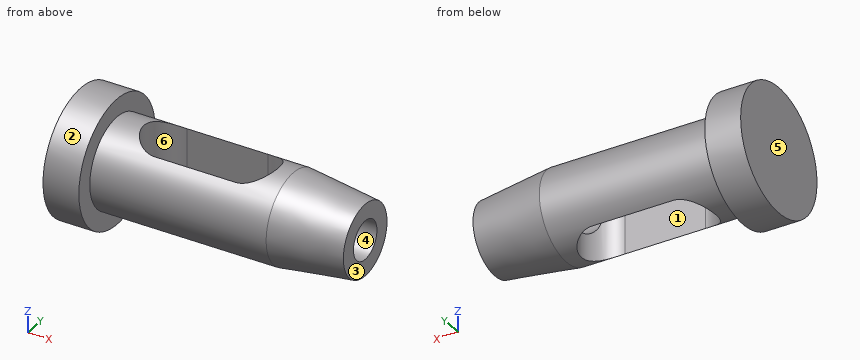
Autodesk Inventor part; units mm, degrees
ref_plane "YZ Plane" through (0, 0, 0) normal (1, 0, 0) x (0, 1, 0)
ref_plane "XZ Plane" through (0, 0, 0) normal (0, 1, 0) x (-1, 0, 0)
ref_plane "XY Plane" through (0, 0, 0) normal (0, 0, 1) x (1, 0, 0)
sketch "Sketch1" plane through (0, 0, 0) normal (0, 0, 1) x (1, 0, 0)
  line L0 (0, 0) -> (-95, 0)
  line L1 (-95, 0) -> (-95, 21)
  line L2 (-95, 21) -> (-83, 21)
  line L3 (-83, 21) -> (-83, 15)
  line L4 (-83, 15) -> (-24, 15)
  line L5 (-24, 15) -> (0, 12)
  line L6 (0, 12) -> (0, 0)
  dimension "d0" = 12
  dimension "d1" = 59
  dimension "d2" = 24
  dimension "d3" = 12
  dimension "d4" = 21
  dimension "d5" = 15
revolve "Revolution1" add sketch "Sketch1" angle 360 about axis through (0, 0, 0) along (-1, 0, 0)
sketch "Sketch2" plane through (0, 0, 0) normal (0, 0, 1) x (1, 0, 0)
  line L0 (-65, 0) -> (-38, 0) construction
  line L1 (-65, -9) -> (-38, -9)
  line L2 (-38, 9) -> (-65, 9)
  arc A0 (-65, 9) -> (-65, -9) centre (-65, 0) ccw
  arc A1 (-38, -9) -> (-38, 9) centre (-38, 0) ccw
  line L3 (-95, -21) -> (-95, 21)
  point P0 (0, 0)
  point P1 (-51.5, 0)
  dimension "d7" = 27
  dimension "d8" = 30
  dimension "d9" = 9
extrude "Extrusion1" cut sketch "Sketch2" against normal through all both and the other way through all
sketch "Sketch3" plane through (0, 0, 0) normal (1, 0, 0) x (0, 0, -1)
  point P0 (0, 0)
  point P1 (0, 0)
hole "Hole1" at (0, 0, 0) direction (-1, 0, 0) diameter 12.9175 depth 40 tip angle 118
properties part number "tool holder"
Verification items for the finished model (mm, model axes). Face numbers are marked on the shaded views. A direction names the side the tool comes from. Give positions to 0.01 mm unless a question says otherwise; leave off trailing zeros. Order: outer loops, then holes, each group sorted by start corner. A loop starts at its lowest first (then second) coordinate and runs counter-clockwise, first axis right, second up. Notation, with made-up numbers: (65, -14) - (104, -14) arc R27 cw to (104, 2) - close; hole circle Ø10 at (19.5, 46.5). An arc over 180 degrees is marked (long way). Answer as CSV lines item,"result". Start each with the question number.
Item 1: Mould release check, pull along Y, two halves, no side actions. Record for the marked faces 1, 2 and 3: released by +Y, released by -Y, zero draft, split by the parting line, or undercut.
Item 2: Material ranges on L1, parallel to Y at x = -37.5, z = 11; L2, parallel to X at y = -5.5, z = -3.5; L3, parallel to Z at x = -23, y = 0 (3 decimals), recorded low to high.
Item 3: Access from +Z, -Z, +X, -X, +Y, -Y to the whole of each face (thin tool, end or side, straight path). Record for the marked faces 4, 5 and 6.
Item 4: Section check B-B, the plane z = 0. Record the boundary of the cut face in (x, y), plus the area to 3 significant figures.
Item 5: Section check A-A, the plane y = 0. Record the boundary of the cut face in (x, z).
Item 6: Gauge pin test, flat ends, axial feed: pin 1 (15 mm diameter, centred on y = 0, z = 0, fed in from +X); pin 2 (2 mm diameter, centred on x = -38, z = 4, fed in from +Y); pin 3 (1 mm diameter, centred on x = -78.5, z = 2, fed in from -Y); pin 4 (10 mm diameter, centred on x = -70.5, z = 14, fed in from +Y). Record the tip position at first contact, or that the pin passes through.
Item 7: Section check D-D, the plane x = -77. Record the boundary of the cut face in (y, z), plus the area to 3 significant figures.
Filled in:
1,face 1,"undercut"
1,face 2,"split by the parting line"
1,face 3,"zero draft"
2,L1,"-10.2 to -8.99, 8.99 to 10.2"
2,L2,"-95 to -72.12, -30.88 to 0"
2,L3,"-14.875 to -6.459, 6.459 to 14.875"
3,face 4,"+X"
3,face 5,"+Z, -Z, -X, +Y, -Y"
3,face 6,"+Z, -Z"
4,outline,"(-95, -21) - (-83, -21) - (-83, -15) - (-24, -15) - (0, -12) - (0, -6.46) - (-31.73, -6.46) arc R9 cw to (-38, -9) - (-65, -9) arc R9 cw to (-65, 9) - (-38, 9) arc R9 cw to (-31.73, 6.46) - (0, 6.46) - (0, 12) - (-24, 15) - (-83, 15) - (-83, 21) - (-95, 21) - close"
4,area,"1,800 mm^2"
5,outline,"(-95, -21) - (-83, -21) - (-83, -15) - (-74, -15) - (-74, 15) - (-83, 15) - (-83, 21) - (-95, 21) - close; (-29, -15) - (-24, -15) - (0, -12) - (0, -6.46) - (-29, -6.46) - close; (-29, 6.46) - (0, 6.46) - (0, 12) - (-24, 15) - (-29, 15) - close"
6,pin 1,"x = 0"
6,pin 2,"y = 14.7"
6,pin 3,"y = -14.92"
6,pin 4,"y = 12"
7,outline,"circle Ø30 at (0, 0)"
7,area,"707 mm^2"
